```python
from build123d import *

# Parameters (mm, degrees)
F0_W     = 124.8
F0_H     = 59.6
F1_DEPTH = 8.1
F2_R     = 10.4
F3_R     = 10.4
F4_T     = -0.5


with BuildPart() as f1:
    # F0 (on Top) → F1 (new body)
    with BuildSketch(Plane.XY):
        with Locations((-62.4, -29.8)):
            Rectangle(F0_W, F0_H)
    extrude(amount=F1_DEPTH)

    # F2
    f2_edges = [f1.edges().sort_by_distance(p)[0] for p in [
        (0, -59.6, 4.05),
    ]]
    fillet(f2_edges, radius=F2_R)

    # F3
    f3_edges = [f1.edges().sort_by_distance(p)[0] for p in [
        (0, 0, 4.05),
        (-124.8, -59.6, 4.05),
        (-124.8, 0, 4.05),
    ]]
    fillet(f3_edges, radius=F3_R)

    # F4
    f4_openings = [f1.faces().sort_by_distance(p)[0] for p in [
        (-62.4, -29.8, 8.1),
    ]]
    offset(amount=F4_T, openings=f4_openings)


solid = f1.part
```
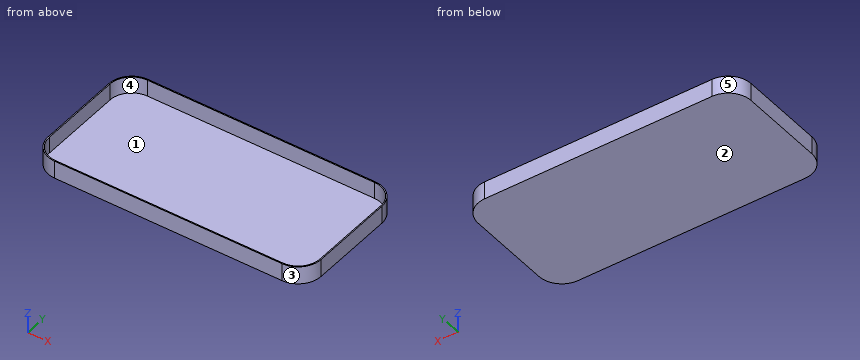
Geometry check sheet. Reference: the model listing, model coordinates, mm. Face numbers are marked on the shaded views. A direction names the side the tool comes from. Round coordinates to 2 decimals unless told otherwise and drop trailing zeros. Loops run counter-clockwise (first coordinate to the right, second up) from the corner with the lowest first, then second, coordinate; pieces in that order, holes last. Notation, with made-up numbers: M 9.5,20 L 54.5,20 A16 cw 54.5,43 Z; hole C 4.5,-18.75 d2. An arc over 180 degrees is marked long. Return JSON: item names as keys, results as strings. Group by question number.
(1) Section check A-A, the plane z = 5.5. Enter the section's corners in (x, y), and give its area (3 significant figures).
(2) Section check B-B, the plane x = -41. Enter the section's corners in (y, z).
(3) Go/stop test with a flat-tipped pin: pin 1 (10 mm diameter, centred on x = -29.5, y = -19, fed in from +Z). Record where the tip stops, or that it passes through.
(4) Set-up check for the marked faces 4 and 5: record each of +Z, -Z, +X, -X, +Y, -Y from which the full face is reachable in a straight line by a thin tool's end or side.
(5) Scan lines: line 1 along Y through (x, z) = (-35, 4.75); line 2 along X through (y, z) = (-16.5, 0.75); line 3 along Z through (x, y) = (-64, -33). Record each from-to range of solid material in increasing order. Write a range as [from, to].
(6) Section check C-C, the plane y = -27. Enter the section's corners in (x, z), and give its area (3 significant figures).
(7) Mould release check, pull along Y, two halves, no side actions. Record for the marked faces 1, 2 and 3: pulls with the +Y half, pulls with the -Y half, needs draft (parallel to the pull), parting line crosses it, or undercut.
Data:
{
 "1": {"outline": "M -124.8,-49.2 A10.4 ccw -114.4,-59.6 L -10.4,-59.6 A10.4 ccw 0,-49.2 L 0,-10.4 A10.4 ccw -10.4,0 L -114.4,0 A10.4 ccw -124.8,-10.4 Z; hole M -124.3,-49.2 A9.9 ccw -114.4,-59.1 L -10.4,-59.1 A9.9 ccw -0.5,-49.2 L -0.5,-10.4 A9.9 ccw -10.4,-0.5 L -114.4,-0.5 A9.9 ccw -124.3,-10.4 Z", "area": "175 mm²"},
 "2": {"outline": "M -59.6,0 L 0,0 L 0,8.1 L -0.5,8.1 L -0.5,0.5 L -59.1,0.5 L -59.1,8.1 L -59.6,8.1 Z"},
 "3": {"pin 1": "z = 0.5"},
 "4": {"face 4": "+Z", "face 5": "+Z, -Z, -X, +Y"},
 "5": {"line 1": "[-59.6, -59.1], [-0.5, 0]", "line 2": "[-124.8, -124.3], [-0.5, 0]", "line 3": "[0, 0.5]"},
 "6": {"outline": "M -124.8,0 L 0,0 L 0,8.1 L -0.5,8.1 L -0.5,0.5 L -124.3,0.5 L -124.3,8.1 L -124.8,8.1 Z", "area": "70.0 mm²"},
 "7": {"face 1": "undercut", "face 2": "needs draft", "face 3": "pulls with the -Y half"}
}
